Can you work these out from the drawing? Everything is in mm from the part's minimum corner. A direction names the side the tool comes from. Give positions to 0.01 mm unless a question says otherwise; leave off trailing zeros. Loops run counter-clockwise (first coordinate to the right, second up) from the corner with the lowest first, then second, coordinate; pieces in that order, holes last. Notation, with made-up numbers: (2.5, -40) - (20.5, -40) arc R27 ccw to (20.5, -6) - close; hole circle Ø8 at (-3, 41). An arc over 180 degrees is marked (long way). One line per item, written item: value. Start each with the question number.
Q1. I want a section at A-A (x = 4). Please give me the cut outline in (y, z), then the cut area to 3 significant figures.
Q2. If I drill on line 1 (X direction, y = 11, z = 10.5), over which ranges is the centre line in solid material (lowest first)? Write a range as from..to.
Q3. For the marked faces 1, 2 and 3, which set-ups out of +Z, -Z, +X, -X, +Y, -Y let a thin tool reach every point of the face, with its end or its side?
Q4. I'm going to push flat-ended pins straight in: P1, Ø12, axis at y = 2.5, z = 12, coming from the -X side; P2, Ø3.5, axis at x = 51.5, y = 7, coming from the -Z side; P3, Ø2, axis at y = 7.5, z = 25.5, coming from the +X side. Where does each tip first touch, or does it pass through?
Q5. I want a section at B-B (z = 20). Please give me the cut outline in (x, y).
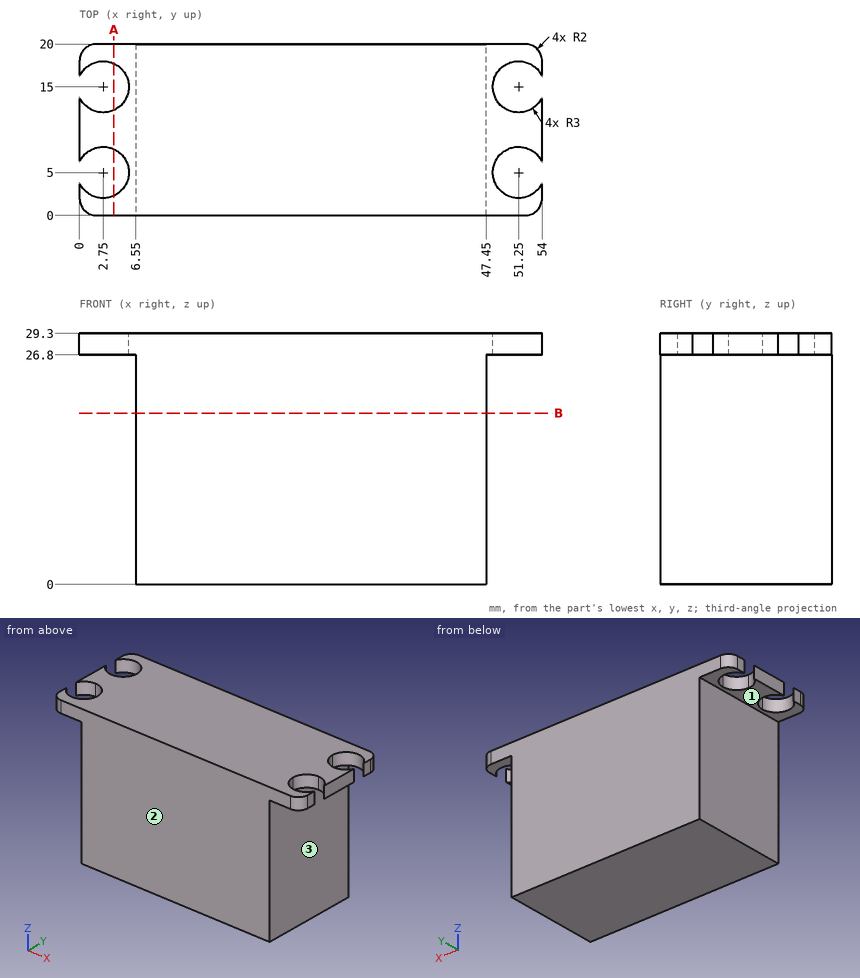
Worked answers:
1. outline: (0, 26.8) - (2.27, 26.8) - (2.27, 29.3) - (0, 29.3) - close; (7.73, 26.8) - (12.27, 26.8) - (12.27, 29.3) - (7.73, 29.3) - close; (17.73, 26.8) - (20, 26.8) - (20, 29.3) - (17.73, 29.3) - close
1. area: 22.7 mm²
2. line 1: x = 6.55..47.45
3. face 1: -Z, -X, +Y, -Y
3. face 2: +Z, -Z, +X, -X, -Y
3. face 3: -Z, +X, +Y, -Y
4. P1: stops at x = 6.55
4. P2: stops at z = 26.8
4. P3: stops at x = 47.45
5. outline: (6.55, 0) - (47.45, 0) - (47.45, 20) - (6.55, 20) - close
